The listing builds one solid part. Answer for the finished solid, in the listing's coordinates (mm). Coordinates: 2 decimals unless noted, no trailing zeros. Write each loop counter-clockwise with the first axis right and the second up, starting at its lowest first coordinate (ties: lowest second). Pieces come first, ordered by that corner, then holes.
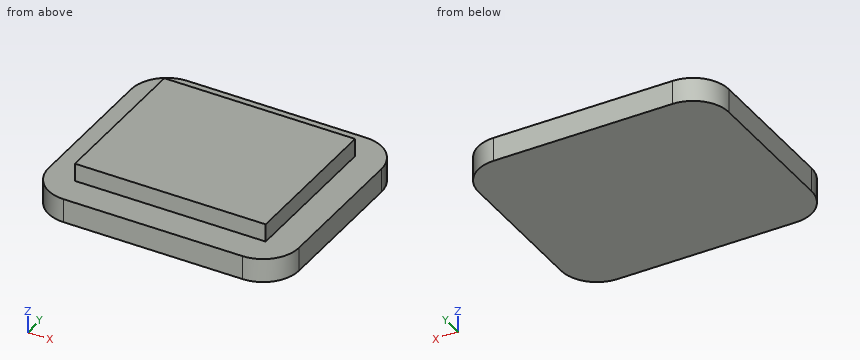
from build123d import *

# Parameters (mm, degrees)
SKETCH_W     = 21
SKETCH_H     = 18
PAD_DEPTH    = 2
SKETCH001_W  = 16
SKETCH001_H  = 13
PAD001_DEPTH = 1.5
FILLET_R     = 3


with BuildPart() as part:
    # Sketch → Pad (new body)
    with BuildSketch(Plane.XY):
        with Locations((-10.5, 9)):
            Rectangle(SKETCH_W, SKETCH_H)
    extrude(amount=PAD_DEPTH)

    # Sketch001 (on Face6 of Pad) → Pad001 (join)
    with BuildSketch(Plane.XY.offset(2)):
        with Locations((-10.5, 9)):
            Rectangle(SKETCH001_W, SKETCH001_H)
    extrude(amount=PAD001_DEPTH)

    # Fillet
    fillet_edges = [part.edges().sort_by_distance(p)[0] for p in [
        (0, 18, 1),
        (0, 0, 1),
        (-21, 0, 1),
        (-21, 18, 1),
    ]]
    fillet(fillet_edges, radius=FILLET_R)


solid = part.part
Q1. Given pin 1 (0.8 mm diameter, centred on y = 11.5, z = 2.5, fed in from +X); pin 2 (0.8 mm diameter, centred on y = 10, z = 3, fed in from -X); pin 3 (1.5 mm diameter, centred on x = -17, z = 3, fed in from +Y); pin 4 (1.6 mm diameter, centred on x = -13, z = 2.5, fed in from -Y), each flat-ended and moving along its own axis, determine where each tip first touches the part or whether it passes through.
Answers below:
pin 1: stops at x = -2.5
pin 2: stops at x = -18.5
pin 3: stops at y = 15.5
pin 4: stops at y = 0
Q2. The part is cut by section A-A, the plane x = -13.5. Write down the section's boundary in (y, z).
Answers below:
outline: (0, 0) - (18, 0) - (18, 2) - (15.5, 2) - (15.5, 3.5) - (2.5, 3.5) - (2.5, 2) - (0, 2) - close
Q3. The part is cut by section C-C, the plane z = 2.85. Write down the section's boundary in (x, y), then the cut area to 3 significant figures.
Answers below:
outline: (-18.5, 2.5) - (-2.5, 2.5) - (-2.5, 15.5) - (-18.5, 15.5) - close
area: 208 mm2
Q4. The part is cut by section B-B, the plane y = 5.25. Write down the section's boundary in (x, z).
Answers below:
outline: (-21, 0) - (0, 0) - (0, 2) - (-2.5, 2) - (-2.5, 3.5) - (-18.5, 3.5) - (-18.5, 2) - (-21, 2) - close
Q5. Find the intervals of material crossed by probe 1 along Z at (x, y) = (-14.75, 1.5); probe 2 along X at (y, z) = (7.25, 2.05); probe 3 along Y at (x, z) = (-9.25, 2.1), in increasing order.
Answers below:
probe 1: z = 0 to 2
probe 2: x = -18.5 to -2.5
probe 3: y = 2.5 to 15.5
Q6. The part is cut by section D-D, the plane x = -1.5. Write down the section's boundary in (y, z), then the cut area to 3 significant figures.
Answers below:
outline: (0.4, 0) - (17.6, 0) - (17.6, 2) - (0.4, 2) - close
area: 34.4 mm2
